from build123d import *

# Parameters (mm, degrees)
F0_W     = 2.5
F0_H     = 2.5
F1_DEPTH = 5
F2_R     = 16.25
F2_W     = 2.5
F2_H     = 2.5
F3_DEPTH = 1
F4_R     = 16.25
F4_W     = 2.5
F4_H     = 2.5
F5_DEPTH = 1
F6_R     = 2.5
F6_W     = 2.5
F6_H     = 2.5
F7_DEPTH = 2.5


with BuildPart() as f1:
    # F0 (on Top) → F1 (new body)
    with BuildSketch(Plane.XY):
        Polygon((16.9110578052, -1.7774237981), (20, 0), (16.9110578052, 1.7774237981), (19.5629520147, 4.1582338164), (16.1719634308, 5.2545894454), (18.2709091529, 8.1347328615), (14.7260766529, 8.5021043196), (16.1803398875, 11.7557050458), (12.6365896616, 11.3780364374), (13.3826121272, 14.8628965095), (9.9948230651, 13.7566937651), (10, 17.3205080757), (6.9162347401, 15.5341175632), (6.1803398875, 19.0211303259), (3.5353737692, 16.6326258829), (2.0905692654, 19.8904379074), (0, 17.0042086393), (-2.0905692654, 19.8904379074), (-3.5353737692, 16.6326258829), (-6.1803398875, 19.0211303259), (-6.9162347401, 15.5341175632), (-10, 17.3205080757), (-9.9948230651, 13.7566937651), (-13.3826121272, 14.8628965095), (-12.6365896616, 11.3780364374), (-16.1803398875, 11.7557050458), (-14.7260766529, 8.5021043196), (-18.2709091529, 8.1347328615), (-16.1719634308, 5.2545894454), (-19.5629520147, 4.1582338164), (-16.9110578052, 1.7774237981), (-20, 0), (-16.9110578052, -1.7774237981), (-19.5629520147, -4.1582338164), (-16.1719634308, -5.2545894454), (-18.2709091529, -8.1347328615), (-14.7260766529, -8.5021043196), (-16.1803398875, -11.7557050458), (-12.6365896616, -11.3780364374), (-13.3826121272, -14.8628965095), (-9.9948230651, -13.7566937651), (-10, -17.3205080757), (-6.9162347401, -15.5341175632), (-6.1803398875, -19.0211303259), (-3.5353737692, -16.6326258829), (-2.0905692654, -19.8904379074), (0, -17.0042086393), (2.0905692654, -19.8904379074), (3.5353737692, -16.6326258829), (6.1803398875, -19.0211303259), (6.9162347401, -15.5341175632), (10, -17.3205080757), (9.9948230651, -13.7566937651), (13.3826121272, -14.8628965095), (12.6365896616, -11.3780364374), (16.1803398875, -11.7557050458), (14.7260766529, -8.5021043196), (18.2709091529, -8.1347328615), (16.1719634308, -5.2545894454), (19.5629520147, -4.1582338164), align=None)
        Rectangle(F0_W, F0_H, mode=Mode.SUBTRACT)
    extrude(amount=F1_DEPTH)

    # F2 (on face) → F3 (cut)
    with BuildSketch(Plane(origin=(0, 0, 0), x_dir=(1, 0, 0), z_dir=(0, 0, -1))):
        Circle(F2_R)
        Rectangle(F2_W, F2_H, mode=Mode.SUBTRACT)
    extrude(amount=-F3_DEPTH, mode=Mode.SUBTRACT)

    # F4 (on face) → F5 (cut)
    with BuildSketch(Plane.XY.offset(5)):
        Circle(F4_R)
        Rectangle(F4_W, F4_H, mode=Mode.SUBTRACT)
    extrude(amount=-F5_DEPTH, mode=Mode.SUBTRACT)

    # F6 (on face) → F7 (join)
    with BuildSketch(Plane(origin=(0, 0, 1), x_dir=(1, 0, 0), z_dir=(0, 0, -1))):
        Circle(F6_R)
        Rectangle(F6_W, F6_H, mode=Mode.SUBTRACT)
    extrude(amount=F7_DEPTH)


solid = f1.part
Read the model definition and answer for the solid it produces. Units are mm, in the model's axes. A direction names the side the tool comes from. Give positions to 0.01 mm unless a question says otherwise; leave off trailing zeros. Write each loop counter-clockwise with the first axis right and the second up, starting at its lowest first coordinate (ties: lowest second). Pieces come first, ordered by that corner, then holes. Notation, with made-up numbers: (2.5, 17.5) -> (61.5, 17.5) arc R12 cw to (61.5, 36.5) -> close; hole circle Ø8 at (-36.5, 49). An arc over 180 degrees is marked (long way). Answer as a JSON object with one key per item and string values. Group by question number.
1) Consider L1, parallel to Z at x = 8.5, y = -2; L2, parallel to Y at x = -8, z = 2; L3, parallel to Z at x = 16.5, y = 5. Determine where each line is inside the solid, lowest interval first. Write a range as from..to.
2) A tool of negligible diameter and unlimited length cuts with its end or side. For faces 4 (the flat face through (17.89, 4.7, 2.46)), 5 (the flat face through (-6.553, -17.253, 2.465)), 6 (the flat face through (0, 1.25, 1)), 7 (the flat face through (-17.844, 4.714, 2.465)), 8 (the cylindrical face through (15.5, 4.88, 4.51)), from which of +Z, -Z, +X, -X, +Y, -Y can it reach the whole face along a straight path? Write none if from no direction.
3) Find section C-C (y = 7.5). Write down the section's boundary in (x, z), and give its area (3 significant figures).
4) Find section A-A (z = 0.5). Count the separate pieces of the cut face and the enclosed holes in it, and give its area (3 significant figures).
5) Each of these flat-tipped pins is pushed along its axis until it touches: P1, Ø0.8, axis at y = 0.5, z = 0.5, coming from the -X side; P2, Ø1, axis at x = -3, y = -2, coming from the +Z side; P3, Ø1.5, axis at y = 7, z = 1.5, coming from the +X side. Where does it stop, or does it pass through?
6) Find section B-B (x = 5). Write down the section's boundary in (y, z), and give its area (3 significant figures).
7) The mould has two halves that part along X. Classify faces 1 (the flat face through (2.9, 16.3, 5)), 2 (the flat face through (-4.876, -17.844, 2.465)), 3 (the flat face through (15.443, 10.106, 2.465)): +X half, -X half, draft (parallel to the pull), parting line (faces both ways), or undercut.
Values follow:
{
 "1": {"L1": "z = 1..4", "L2": "y = -16.16..16.16", "L3": "z = 0..5"},
 "2": {"face 4": "+Z, -Z, +X", "face 5": "+Z, -Z, -Y", "face 6": "+Z, -Z", "face 7": "+Z, -Z, -X", "face 8": "+Z"},
 "3": {"outline": "(-17.81, 0) -> (-14.42, 0) -> (-14.42, 1) -> (14.42, 1) -> (14.42, 0) -> (17.81, 0) -> (17.81, 5) -> (14.42, 5) -> (14.42, 4) -> (-14.42, 4) -> (-14.42, 5) -> (-17.81, 5) -> close", "area": "120 mm2"},
 "4": {"separate pieces": "2", "enclosed holes": "2", "area": "250 mm2"},
 "5": {"P1": "stops at x = -19.83", "P2": "stops at z = 4", "P3": "stops at x = 17.99"},
 "6": {"outline": "(-17.96, 0) -> (-15.46, 0) -> (-15.46, 1) -> (15.46, 1) -> (15.46, 0) -> (17.96, 0) -> (17.96, 5) -> (15.46, 5) -> (15.46, 4) -> (-15.46, 4) -> (-15.46, 5) -> (-17.96, 5) -> close", "area": "118 mm2"},
 "7": {"face 1": "draft", "face 2": "undercut", "face 3": "+X half"}
}
